Can you work these out from the drawing? Everything is in mm from the part's minimum corner. A direction names the side the tool comes from. Round coordinates to 2 decimals unless told otherwise and drop trailing zeros. Loops run counter-clockwise (first coordinate to the right, second up) from the corner with the lowest first, then second, coordinate; pieces in that order, holes last. Notation, with made-up numbers: (1.5, 58) -> (25.5, 58) arc R9 ccw to (25.5, 70) -> close; hole circle Ø7 at (9.5, -28.5). An arc over 180 degrees is marked (long way). One line per item, written item: value.
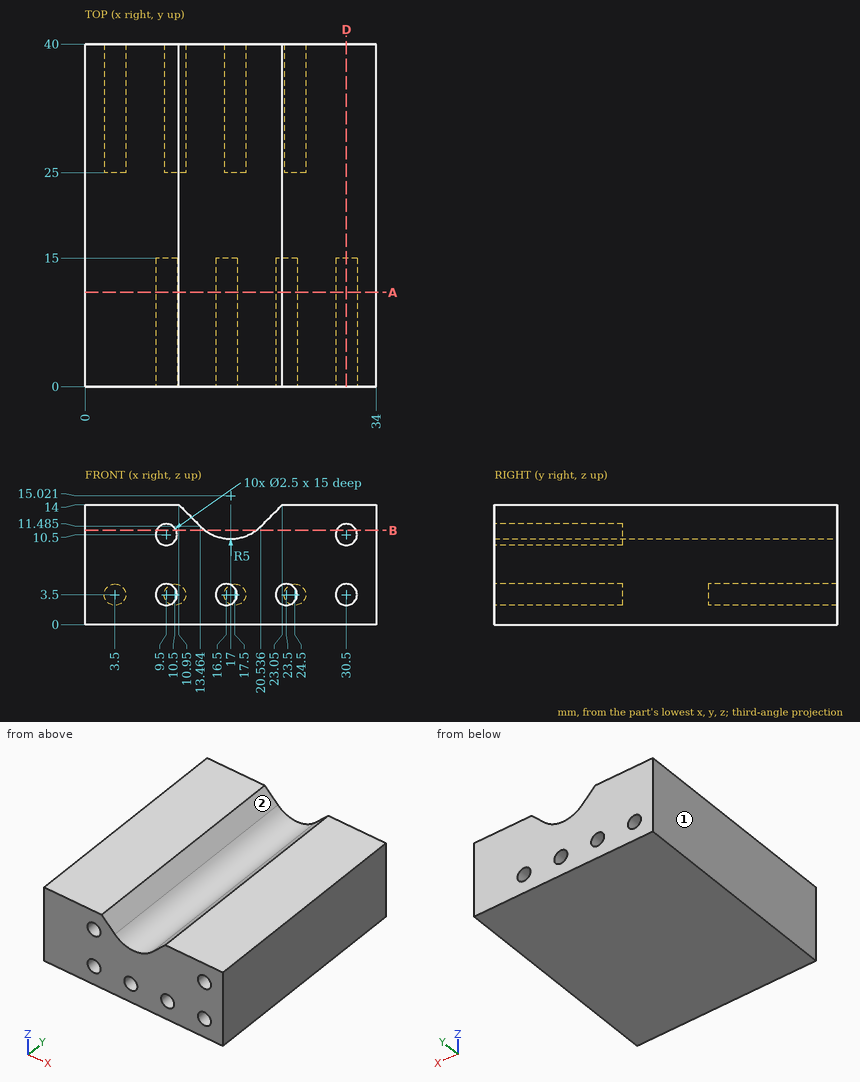
(1) For pin 1 Ø1.2 at (x, z) = (9.5, 11) entering from -Y; pin 2 Ø0.8 at (x, z) = (24.5, 3.5) entering from +Y, each with a flat end and sliding along its axis, tell me the tip position at first contact or that it passes through.
Results below:
pin 1: stops at y = 15
pin 2: stops at y = 25
(2) On a 3-axis mill with a long thin cutter (end or side, diameter ignored), from which of +Z, -Z, +X, -X, +Y, -Y can I reach the whole of each face in a straight line? I mean the marked faces 1 and 2. Say none if no direction works.
Results below:
face 1: +Z, -Z, -X, +Y, -Y
face 2: +Z, +Y, -Y
(3) Please list where these lines run through material, in increasing order: L1, parallel to X at y = 35.5, z = 3.5; L2, parallel to X at y = 7, z = 3.5; L3, parallel to Z at x = 10.5, y = 10.
Results below:
L1: x = 0 to 2.25, 4.75 to 9.25, 11.75 to 16.25, 18.75 to 23.25, 25.75 to 34
L2: x = 0 to 8.25, 10.75 to 15.25, 17.75 to 22.25, 24.75 to 29.25, 31.75 to 34
L3: z = 0 to 2.75, 4.25 to 9.75, 11.25 to 14
(4) Imagine slicing it at A-A on y = 11. Give the number of separate pieces and of enclosed holes in the cut face, then the cut area to 3 significant figures.
Results below:
separate pieces: 1
enclosed holes: 6
area: 415 mm²
(5) Imagine slicing it at D-D on x = 30.5. Write out the boundary of the cut face in (y, z).
Results below:
outline: (0, 0) -> (40, 0) -> (40, 14) -> (0, 14) -> (0, 11.75) -> (15, 11.75) -> (15, 9.25) -> (0, 9.25) -> (0, 4.75) -> (15, 4.75) -> (15, 2.25) -> (0, 2.25) -> close
(6) Imagine slicing it at B-B on z = 11. Write out the boundary of the cut face in (x, y) (1 decimal).
Results below:
outline: (0, 0) -> (8.4, 0) -> (8.4, 15) -> (10.6, 15) -> (10.6, 0) -> (14, 0) -> (14, 40) -> (0, 40) -> close; (20, 0) -> (29.4, 0) -> (29.4, 15) -> (31.6, 15) -> (31.6, 0) -> (34, 0) -> (34, 40) -> (20, 40) -> close
